```python
from build123d import *

# Parameters (mm, degrees)
F0_W      = 50.00625
F0_H      = 37.30625
F0_R      = 1.984375
F0_W_2    = 19.05
F0_H_2    = 5.55625
F1_DEPTH  = 6.35
F2_W      = 7.9375
F2_H      = 5.55625
F2_H_2    = 11.1125
F3_DEPTH  = 4.7625
F5_R      = 1.984375
F6_R      = 2.778125
F8_R      = 2.778125
F9_R      = 1.984375
F11_W     = 19.05
F11_H     = 6.35
F12_DEPTH = 25.4


with BuildPart() as f1:
    # F0 (on Top) → F1 (new body)
    with BuildSketch(Plane.XY):
        Rectangle(F0_W, F0_H)
        with Locations((0, -5.953125)):
            Circle(F0_R, mode=Mode.SUBTRACT)
        with Locations((0, 5.953125)):
            Rectangle(F0_W_2, F0_H_2, mode=Mode.SUBTRACT)
        with Locations((0, 12.303125)):
            Circle(F0_R, mode=Mode.SUBTRACT)
    extrude(amount=F1_DEPTH)

    # F2 (on face) → F3 (cut)
    with BuildSketch(Plane.XY.offset(6.35)):
        Polygon((-3.175, 14.684375), (-23.415625, 14.684375), (-23.415625, 9.128125), (-25.003125, 9.128125), (-25.003125, 2.778125), (-23.415625, 2.778125), (0, 2.778125), (23.415625, 2.778125), (25.003125, 2.778125), (25.003125, 9.128125), (23.415625, 9.128125), (23.415625, 14.684375), (3.175, 14.684375), (3.175, 9.128125), (-3.175, 9.128125), align=None)
        with Locations((-19.446875, -1.5875)):
            Rectangle(F2_W, F2_H)
        Polygon((-0.79375, 1.190625), (-13.890625, 1.190625), (-13.890625, -4.365625), (-3.175, -4.365625), (-3.175, -2.778125), (-0.79375, -2.778125), align=None)
        with Locations((-19.446875, -11.509375)):
            Rectangle(F2_W, F2_H_2)
        Polygon((-3.175, -5.953125), (-13.890625, -5.953125), (-13.890625, -17.065625), (-0.79375, -17.065625), (-0.79375, -9.128125), (-3.175, -9.128125), align=None)
        Polygon((0.79375, -2.778125), (3.175, -2.778125), (3.175, -4.365625), (13.890625, -4.365625), (13.890625, 1.190625), (0.79375, 1.190625), align=None)
        Polygon((13.890625, -5.953125), (3.175, -5.953125), (3.175, -9.128125), (0.79375, -9.128125), (0.79375, -17.065625), (13.890625, -17.065625), align=None)
        with Locations((19.446875, -1.5875)):
            Rectangle(F2_W, F2_H)
        with Locations((19.446875, -11.509375)):
            Rectangle(F2_W, F2_H_2)
    extrude(amount=-F3_DEPTH, mode=Mode.SUBTRACT)

    # F5 (on offset) → F7 section 0
    with BuildSketch(Plane(origin=(0, 0, 1.5875), x_dir=(1, 0, 0), z_dir=(0, 0, -1))):
        with Locations((0, -12.303125)):
            Circle(F5_R)
    # F6 (on face) → F7 section 1
    with BuildSketch(Plane(origin=(0, 0, 0), x_dir=(1, 0, 0), z_dir=(0, 0, -1))):
        with Locations((0, -12.303125)):
            Circle(F6_R)
    loft(mode=Mode.SUBTRACT)

    # F8 (on face) → F10 section 0
    with BuildSketch(Plane(origin=(0, 0, 0), x_dir=(1, 0, 0), z_dir=(0, 0, -1))):
        with Locations((0, 5.953125)):
            Circle(F8_R)
    # F9 (on offset) → F10 section 1
    with BuildSketch(Plane(origin=(0, 0, 1.5875), x_dir=(1, 0, 0), z_dir=(0, 0, -1))):
        with Locations((0, 5.953125)):
            Circle(F9_R)
    loft(mode=Mode.SUBTRACT)

    # F11 (on face) → F12 (cut)
    with BuildSketch(Plane.XY.offset(1.5875)):
        with Locations((0, 5.953125)):
            Rectangle(F11_W, F11_H)
    extrude(amount=-F12_DEPTH, mode=Mode.SUBTRACT)


solid = f1.part
```
Geometry: final body of the model. Coordinates: model frame, mm. A direction names the side the tool comes from. Coordinates: 2 decimals unless noted, no trailing zeros. Order: outer loops, then holes, each group sorted by start corner. A loop starts at its lowest first (then second) coordinate and runs counter-clockwise, first axis right, second up. Notation, with made-up numbers: M -32,85 L 4,85 A17 cw 4,111 Z; hole C -25,72.25 d6. An arc over 180 degrees is marked long. Answer as CSV lines item,"result".
Q1. Line query: probe 1 along Y at (x, z) = (-16, 5.5); probe 2 along Y at (x, z) = (3, 4); probe 3 along X at (y, z) = (-10, 2). Output: solid intervals per line, ascending. Write a range as [from, to].
Answers:
probe 1,"y = [-18.65, -17.07], [-5.95, -4.37], [1.19, 2.78], [14.68, 18.65]"
probe 2,"y = [-18.65, -17.07], [-9.13, -2.78], [1.19, 2.78], [9.13, 18.65]"
probe 3,"x = [-25, -23.42], [-15.48, -13.89], [-0.79, 0.79], [13.89, 15.48], [23.42, 25]"
Q2. Section B-B on y = 4. Return the cut outline in (x, z) (1 decimal), and give its area (3 significant figures).
Answers:
outline,"M -25,0 L -9.5,0 L -9.5,1.6 L -25,1.6 Z; M 9.5,0 L 25,0 L 25,1.6 L 9.5,1.6 Z"
area,"49.1 mm^2"
Q3. Section D-D on x = 18. Return the cut outline in (y, z), and give its area (3 significant figures).
Answers:
outline,"M -18.65,0 L 18.65,0 L 18.65,6.35 L 14.68,6.35 L 14.68,1.59 L 2.78,1.59 L 2.78,6.35 L 1.19,6.35 L 1.19,1.59 L -4.37,1.59 L -4.37,6.35 L -5.95,6.35 L -5.95,1.59 L -17.07,1.59 L -17.07,6.35 L -18.65,6.35 Z"
area,"101 mm^2"
Q4. Set-up query: faces 5 (the flat face through (0, 0, 0)), 6 (the flat face through (-13.891, -2, 4)). Return all of +Z, -Z, +X, -X, +Y, -Y with unobstructed straight access to the full face (end or side cutting, diameter ignored); none if empty.
Answers:
face 5,"-Z, +X, -X, +Y, -Y"
face 6,"+Z"
Q5. Section A-A on x = -7. Return the cut outline in (y, z), and give its area (3 significant figures).
Answers:
outline,"M -18.65,0 L 2.78,0 L 2.78,6.35 L 1.19,6.35 L 1.19,1.59 L -4.37,1.59 L -4.37,6.35 L -5.95,6.35 L -5.95,1.59 L -17.07,1.59 L -17.07,6.35 L -18.65,6.35 Z; M 9.13,0 L 18.65,0 L 18.65,6.35 L 14.68,6.35 L 14.68,1.59 L 9.13,1.59 Z"
area,"90.7 mm^2"
Q6. Draft query along X for faces 1 (the flat face through (-23.416, -12, 4)), 2 (the flat face through (-25.003, 0, 3)), 3 (the flat face through (-7, -2, 1.587)), 4 (the flat face through (-24, 9.128, 4)). Return one class per face: pulls with the +X half, pulls with the -X half, needs draft (parallel to the pull), parting line crosses it, or undercut.
Answers:
face 1,"undercut"
face 2,"pulls with the -X half"
face 3,"undercut"
face 4,"needs draft"
Q7. Section C-C on x = 0. Count the separate pieces of the cut face and the enclosed holes in it, and give its area (3 significant figures).
Answers:
separate pieces,"4"
enclosed holes,"0"
area,"144 mm^2"
Q8. First-contact query: P1, Ø3, axis at x = 5, y = -0.5, coming from the +Z side. Flat tip, straight axial feed; report the tip coordinate or a pass-through.
Answers:
P1,"stops at z = 1.59"
